Verification items for the finished model (mm, model axes). Face numbers are marked on the shaded views. A direction names the side the tool comes from. Give positions to 0.01 mm unless a question says otherwise; leave off trailing zeros. Write each loop counter-clockwise with the first axis right and the second up, starting at its lowest first coordinate (ties: lowest second). Pieces come first, ordered by that corner, then holes. Notation, with made-up numbers: M -4.75,62 L 5.25,62 A22 cw 5.25,79 Z; hole C 10,75 d2. An arc over 180 degrees is marked long. Write item = value, one per line.
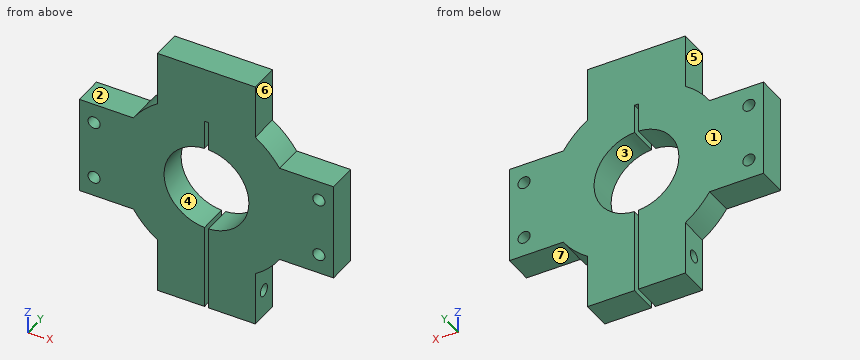
from build123d import *

# Parameters (mm, degrees)
F1_DEPTH = 15
F2_R     = 3.1
F3_DEPTH = 25
F4_R     = 3.1
F5_DEPTH = 56.6


with BuildPart() as f1:
    # F0 (on Front) → F1 (new body)
    with BuildSketch(Plane.XZ):
        with BuildLine():
            Line((65, 25), (37.416574, 25))
            ThreePointArc((37.416574, 25), (31.819805, 31.819805), (25, 37.416574))
            Line((25, 37.416574), (25, 65))
            Line((25, 65), (1, 65))
            Line((1, 65), (-1, 65))
            Line((-1, 65), (-25, 65))
            Line((-25, 65), (-25, 37.416574))
            ThreePointArc((-25, 37.416574), (-31.819805, 31.819805), (-37.416574, 25))
            Line((-37.416574, 25), (-65, 25))
            Line((-65, 25), (-65, -25))
            Line((-65, -25), (-37.416574, -25))
            ThreePointArc((-37.416574, -25), (-31.819805, -31.819805), (-25, -37.416574))
            Line((-25, -37.416574), (-25, -65))
            Line((-25, -65), (-1, -65))
            Line((-1, -65), (-1, -21.676946))
            ThreePointArc((-1, -21.676946), (-21.7, 0), (-1, 21.676946))
            Line((-1, 21.676946), (-1, 36.615141))
            Line((-1, 36.615141), (1, 36.615141))
            Line((1, 36.615141), (1, 21.676946))
            ThreePointArc((1, 21.676946), (21.7, 0), (1, -21.676946))
            Line((1, -21.676946), (1, -65))
            Line((1, -65), (25, -65))
            Line((25, -65), (25, -37.416574))
            ThreePointArc((25, -37.416574), (31.819805, -31.819805), (37.416574, -25))
            Line((37.416574, -25), (65, -25))
            Line((65, -25), (65, 25))
        make_face()
    extrude(amount=F1_DEPTH)

    # F2 (on face) → F3 (cut)
    with BuildSketch(Plane.XZ.offset(15)):
        with Locations((57.5, 15)):
            Circle(F2_R)
        with Locations((57.5, -15)):
            Circle(F2_R)
        with Locations((-57.5, 15)):
            Circle(F2_R)
        with Locations((-57.5, -15)):
            Circle(F2_R)
    extrude(amount=-F3_DEPTH, mode=Mode.SUBTRACT)

    # F4 (on face) → F5 (cut)
    with BuildSketch(Plane(origin=(-25, 0, 0), x_dir=(0, -1, 0), z_dir=(-1, 0, 0))):
        with Locations((7.5, -51.208287)):
            Circle(F4_R)
    extrude(amount=-F5_DEPTH, mode=Mode.SUBTRACT)


solid = f1.part
1) Cross-section at B-B on y = -7.5. Count the separate pieces of the cut face and the enclosed holes in it, plus the area to 3 significant figures.
From the geometry:
separate_pieces = 3
enclosed_holes = 4
area = 8,830 mm^2
2) Tool access check on the marked faces 5, 6 and 7. Record the directions out of +Z, -Z, +X, -X, +Y, -Y that give a thin tool (end or side, any length) a straight path to the whole face; none if there is none.
From the geometry:
face_5 = +Z, -X, +Y, -Y
face_6 = +Z, +X, +Y, -Y
face_7 = -Z, +X, +Y, -Y
3) Cross-section at A-A on x = -57.5. Record the boundary of the cut face in (y, z).
From the geometry:
outline = M -15,-25 L 0,-25 L 0,-18.1 L -15,-18.1 Z; M -15,-11.9 L 0,-11.9 L 0,11.9 L -15,11.9 Z; M -15,18.1 L 0,18.1 L 0,25 L -15,25 Z
4) Depth check by flat-ended pin: P1, Ø7.5, axis at y = -7, z = 31.5, coming from the +X side; P2, Ø8, axis at y = -11.5, z = -48, coming from the -X side; P3, Ø4.5, axis at x = 49, y = -10.5, coming from the -Z side. Enter the tip coordinate at first touch or a pass-through.
From the geometry:
P1 = 35.43
P2 = -25
P3 = -25
5) Cross-section at D-D on x = 46.5. Record the boundary of the cut face in (y, z), plus the area to 3 significant figures.
From the geometry:
outline = M -15,-25 L 0,-25 L 0,25 L -15,25 Z
area = 750 mm^2
6) Cross-section at C-C on z = 15. Record the boundary of the cut face in (x, y), plus the area to 3 significant figures.
From the geometry:
outline = M -65,-15 L -60.6,-15 L -60.6,0 L -65,0 Z; M -54.4,-15 L -15.68,-15 L -15.68,0 L -54.4,0 Z; M 15.68,-15 L 54.4,-15 L 54.4,0 L 15.68,0 Z; M 60.6,-15 L 65,-15 L 65,0 L 60.6,0 Z
area = 1,290 mm^2
7) Draft check along Z on the marked faces 1, 2, 3 and 4. Enter one of: +Z half, -Z half, draft (parallel to the pull), parting line (faces both ways), or undercut.
From the geometry:
face_1 = draft
face_2 = +Z half
face_3 = undercut
face_4 = undercut
8) Material ranges on probe 1 along Z at (x, y) = (-57.5, -9.75); probe 2 along Z at (x, y) = (8, -7.5); probe 3 along Z at (x, y) = (-53, -1), recorded low to high. Write a range as from..to.
From the geometry:
probe_1 = -25..-18.1, -11.9..11.9, 18.1..25
probe_2 = -65..-54.31, -48.11..-20.17, 20.17..65
probe_3 = -25..25
